The listing builds one solid part. Answer for the finished solid, in the listing's coordinates (mm). A direction names the side the tool comes from. Give positions to 0.01 mm unless a question says otherwise; leave off trailing zeros. Write each loop counter-clockwise with the first axis right and the second up, starting at its lowest first coordinate (ties: lowest second). Pieces come first, ordered by that corner, then holes.
```python
from build123d import *

# Parameters (mm, degrees)
PAD_DEPTH       = 4
PAD001_DEPTH    = 2
SKETCH002_R     = 3
SKETCH002_R_2   = 1.25
POCKET_DEPTH    = 2.001
PAD002_DEPTH    = 13
CHAMFER_SIZE    = 0.6
CHAMFER001_SIZE = 0.6
CHAMFER002_SIZE = 0.6
CHAMFER003_SIZE = 0.6
FILLET_R        = 1


with BuildPart() as part:
    # Sketch → Pad (new body)
    with BuildSketch(Plane.XY):
        with BuildLine():
            ThreePointArc((0, 10), (-10, 0), (0, -10))
            Line((0, -10), (19, -10))
            ThreePointArc((19, -10), (29, 0), (19, 10))
            Line((0, 10), (19, 10))
        make_face()
        with BuildLine():
            Line((9, 3.9), (24, 3.9))
            ThreePointArc((24, -3.9), (27.9, 0), (24, 3.9))
            Line((9, -3.9), (24, -3.9))
            ThreePointArc((9, -3.9), (7.389325, -4.156777), (5.938336, -4.90165))
            ThreePointArc((5.938336, 4.90165), (-7.7, 0), (5.938336, -4.90165))
            ThreePointArc((5.938336, 4.90165), (7.389325, 4.156777), (9, 3.9))
        make_face(mode=Mode.SUBTRACT)
    extrude(amount=PAD_DEPTH)

    # Sketch001 → Pad001 (join)
    with BuildSketch(Plane.XY):
        with BuildLine():
            ThreePointArc((0, 10), (-10, 0), (0, -10))
            Line((0, -10), (19, -10))
            ThreePointArc((19, -10), (29, 0), (19, 10))
            Line((0, 10), (19, 10))
        make_face()
    extrude(amount=-PAD001_DEPTH)

    # Sketch002 → Pocket (cut, through all)
    with BuildSketch(Plane.XY):
        Circle(SKETCH002_R)
        with Locations((24, 0)):
            Circle(SKETCH002_R_2)
        with Locations((20, 0)):
            Circle(SKETCH002_R_2)
    extrude(amount=-POCKET_DEPTH, mode=Mode.SUBTRACT)

    # Sketch003 → Pad002 (join)
    with BuildSketch(Plane.XY.offset(-2)):
        with BuildLine():
            ThreePointArc((0, 10), (-10, 0), (0, -10))
            Line((0, -10), (19, -10))
            ThreePointArc((19, -10), (29, 0), (19, 10))
            Line((0, 10), (19, 10))
        make_face()
        with BuildLine():
            Line((-7, -1.427009), (-7, 1.427009))
            Line((-7, 1.427009), (-3.195879, 1.427009))
            ThreePointArc((3.160298, 1.504166), (-0.042483, 3.499742), (-3.195879, 1.427009))
            Line((3.160298, 1.504166), (16.293582, 1.504166))
            ThreePointArc((22.000011, 3.464103), (18.700656, 3.783088), (16.293582, 1.504166))
            ThreePointArc((22.000011, -3.464103), (27.999995, 0), (22.000011, 3.464103))
            ThreePointArc((16.290212, -1.495834), (18.696407, -3.781626), (22.000011, -3.464103))
            Line((3.16425, -1.495834), (16.290212, -1.495834))
            ThreePointArc((-3.195879, -1.427009), (-0.037873, -3.499795), (3.16425, -1.495834))
            Line((-3.195879, -1.427009), (-7, -1.427009))
        make_face(mode=Mode.SUBTRACT)
    extrude(amount=-PAD002_DEPTH)

    # Chamfer
    chamfer_edges = [part.edges().sort_by_distance(p)[0] for p in [
        (9.727231, -1.495834, -15),
        (9.72694, 1.504166, -15),
    ]]
    chamfer(chamfer_edges, length=CHAMFER_SIZE)

    # Chamfer001
    chamfer001_edges = [part.edges().sort_by_distance(p)[0] for p in [
        (19.018709, -3.877772, -15),
        (27.999995, 0, -15),
        (19.023455, 3.87897, -15),
        (-0.392985, 3.477868, -15),
        (-0.387811, -3.478448, -15),
    ]]
    chamfer(chamfer001_edges, length=CHAMFER001_SIZE)

    # Chamfer002
    chamfer002_edges = [part.edges().sort_by_distance(p)[0] for p in [
        (-5.421825, -1.427009, -15),
    ]]
    chamfer(chamfer002_edges, length=CHAMFER002_SIZE)

    # Chamfer003
    chamfer003_edges = [part.edges().sort_by_distance(p)[0] for p in [
        (-5.421825, 1.427009, -15),
        (-7, 0, -15),
        (-7, -1.727009, -15),
    ]]
    chamfer(chamfer003_edges, length=CHAMFER003_SIZE)

    # Fillet
    fillet_edges = [part.edges().sort_by_distance(p)[0] for p in [
        (9.5, 10, -15),
        (29, 0, -15),
        (9.5, -10, -15),
        (-10, 0, -15),
    ]]
    fillet(fillet_edges, radius=FILLET_R)


solid = part.part
```
Item 1: A cutting plane is placed at C-C, the plane x = 4.5. Give the vertices of the cut face in (y, z).
Conclusion:
outline: (-10, -14) arc R1 ccw to (-9, -15) - (-2.1, -15) - (-1.5, -14.4) - (-1.5, -2) - (1.5, -2) - (1.5, -14.4) - (2.1, -15) - (9, -15) arc R1 ccw to (10, -14) - (10, 4) - (6.25, 4) - (6.25, 0) - (-6.25, 0) - (-6.25, 4) - (-10, 4) - close
Item 2: A cutting plane is placed at A-A, the plane y = 0. Count the separate pieces of the cut face and the enclosed holes in it, plus the area to 3 significant figures.
Conclusion:
separate pieces: 4
enclosed holes: 0
area: 121 mm2
Item 3: Each of these flat-tipped pins is pushed along its axis until it touches: P1, Ø4, axis at x = -5.5, z = -9, coming from the +Y side; P2, Ø1, axis at x = -1.5, z = -0.5, coming from the +Y side; P3, Ø8, axis at x = 0, y = 0, coming from the +Z side. Where does it stop, or does it pass through?
Conclusion:
P1: stops at y = 9.37
P2: stops at y = 9.95
P3: stops at z = 0
Item 4: Consider probe 1 along Y at (x, z) = (15, -11); probe 2 along Y at (x, z) = (8, 2); probe 3 along X at (y, z) = (0, 1.65). Determine where each line is inside the solid, lowest interval first.
Conclusion:
probe 1: y = -10 to -1.5, 1.5 to 10
probe 2: y = -10 to -4, 4 to 10
probe 3: x = -10 to -7.7, 27.9 to 29
Item 5: Which of the six approach directions +Z, -Z, +X, -X, +Y, -Y give full straight-line access (tool end or side, diameter ignored) to faces 5 (the face through (14, 0, -2)), 6 (the face through (7.368, 4.164, 1.972)), 7 (the face through (21.155, -0.479, -0.986))?
Conclusion:
face 5: -Z
face 6: +Z
face 7: +Z, -Z
Item 6: Determine the mould class of faces 1 (the face through (29, 0, -5)), 2 (the face through (18.7, 3.95, -14.56)), 3 (the face through (-10, 0, -5)), 4 (the face through (-5, 1.427, -8)) for opening direction X: pulls with the +X half, pulls with the -X half, needs draft (parallel to the pull), parting line crosses it, or undercut.
Conclusion:
face 1: pulls with the +X half
face 2: undercut
face 3: pulls with the -X half
face 4: undercut
Item 7: A cutting plane is placed at B-B, the plane x = 13.5. Give the vertices of the cut face in (y, z).
Conclusion:
outline: (-10, -14) arc R1 ccw to (-9, -15) - (-2.1, -15) - (-1.5, -14.4) - (-1.5, -2) - (1.5, -2) - (1.5, -14.4) - (2.1, -15) - (9, -15) arc R1 ccw to (10, -14) - (10, 4) - (3.9, 4) - (3.9, 0) - (-3.9, 0) - (-3.9, 4) - (-10, 4) - close
